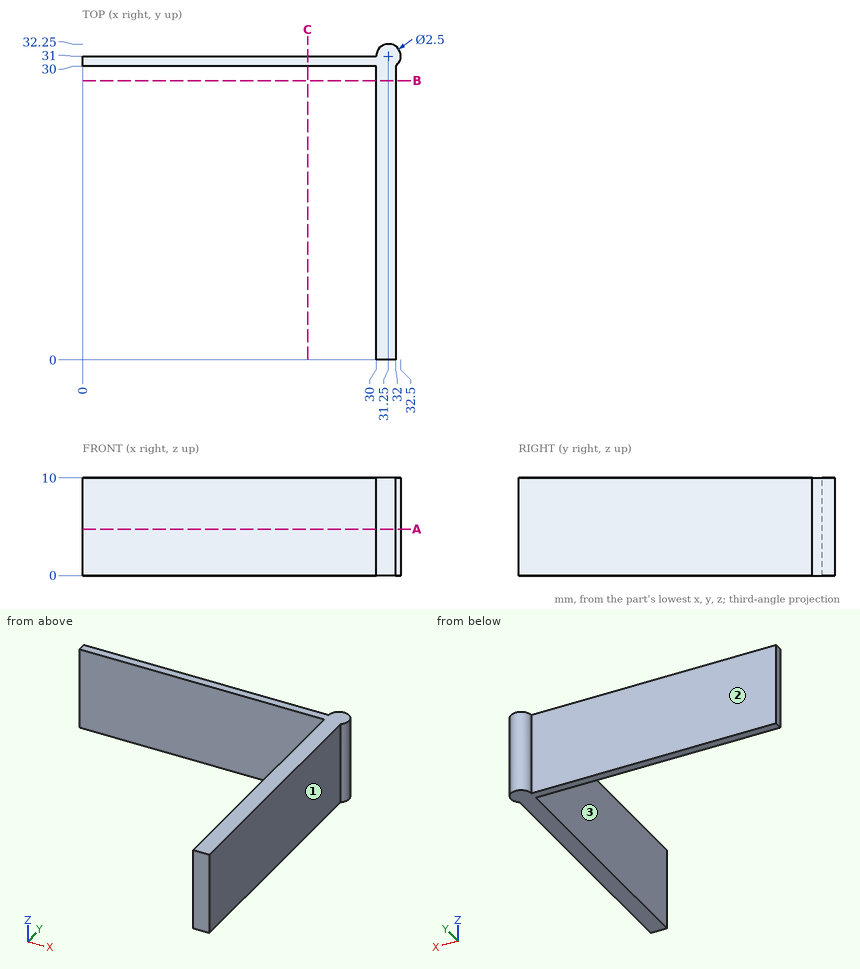
Design review of the part shown in the three views and the two pictorial views. Dimensions are in mm from the part's minimum x, y and z. A direction names the side the tool comes from. Coordinates: 2 decimals unless noted, no trailing zeros. Loops run counter-clockwise (first coordinate to the right, second up) from the corner with the lowest first, then second, coordinate; pieces in that order, holes last.
Q1. We need section A-A on z = 4.75. State the section outline as (x, y) points.
Reported:
outline: (0, 30) - (30, 30) - (30, 0) - (32, 0) - (32, 30) arc R1.25 ccw (long way) to (30, 31) - (0, 31) - close
Q2. Tool access review of the marked faces 1, 2 and 3: name each direction out of +Z, -Z, +X, -X, +Y, -Y from which nothing blocks a thin tool from reaching the whole face with its end or side.
Reported:
face 1: +Z, -Z, +X, -Y
face 2: +Z, -Z, -X, +Y
face 3: +Z, -Z, -X, -Y
Q3. We need section C-C on x = 23. State the section outline as (y, z) points.
Reported:
outline: (30, 0) - (31, 0) - (31, 10) - (30, 10) - close
Q4. To check wall thickness, follow line 1 (Y direction, x = 21, z = 2.5); line 2 (X direction, y = 11, z = 5.5); line 3 (X direction, y = 30.5, z = 6). State the ranges of each line that lie inside material, in increasing order.
Reported:
line 1: y = 30 to 31
line 2: x = 30 to 32
line 3: x = 0 to 32.4
Q5. We need section B-B on y = 28.5. State the section outline as (x, z) points, and give its area (3 significant figures).
Reported:
outline: (30, 0) - (32, 0) - (32, 10) - (30, 10) - close
area: 20.0 mm2
Q6. For pin 1 (3 mm diameter, centred on y = 17.5, z = 5, fed in from -X); pin 2 (1.5 mm diameter, centred on y = 23, z = 3.5, fed in from +X); pin 3 (10 mm diameter, centred on x = 13.5, y = 20.5, fed in from +Z), all flat-tipped, find the tip position at first contact; note any pin that passes through.
Reported:
pin 1: stops at x = 30
pin 2: stops at x = 32
pin 3: passes through
